Here's the drawing with two shaded views (mm, measured from the low corner). I have some questions. Give positions to 0.01 mm unless a question says otherwise; leave off trailing zeros. Loops run counter-clockwise (first coordinate to the right, second up) from the corner with the lowest first, then second, coordinate; pieces in that order, holes last. Notation, with made-up numbers: (60, 18.5) - (97, 18.5) arc R13 ccw to (97, 28.5) - close; hole circle Ø1 at (26.25, -5.75). An arc over 180 degrees is marked (long way). Use a Markdown table: item, result. Add a question column.
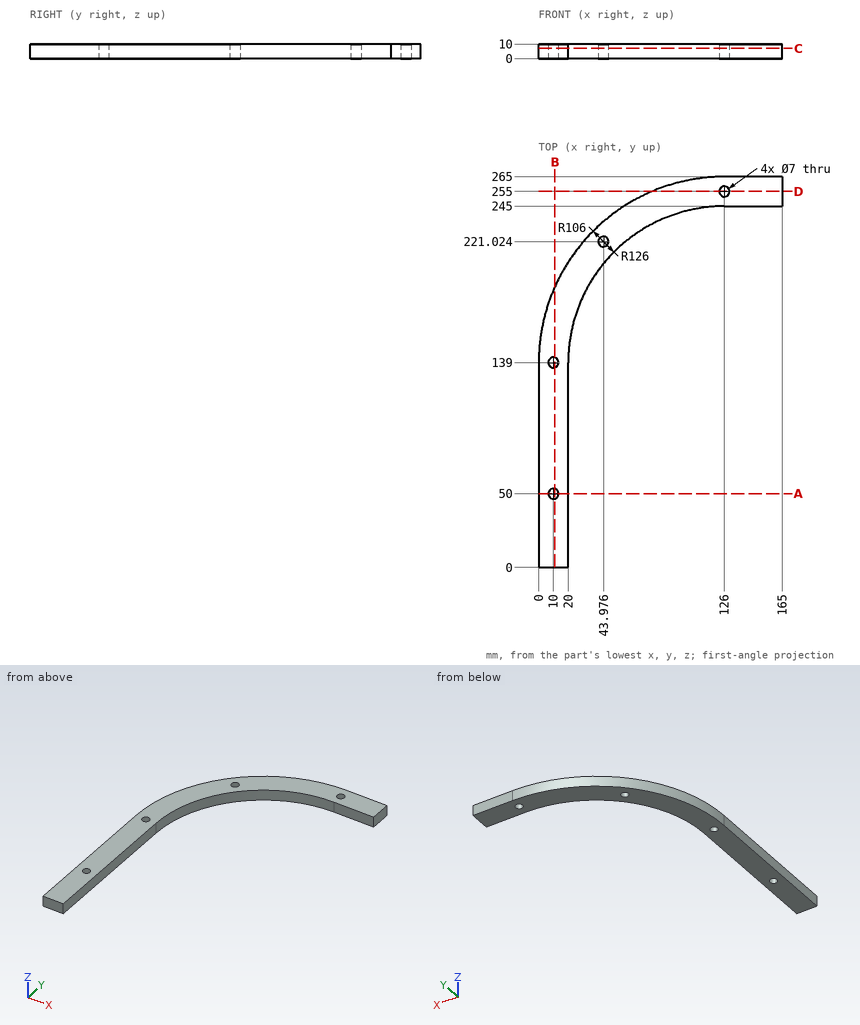
1. Suppose I cut it at B-B (x = 11). List the corners of the cut face in (y, z) for me, and give its area (3 significant figures).
2. Will these pins go through, and if not, where does the flat tip stop? P1, Ø11, axis at x = 126, y = 255, coming from the +Z side; P2, Ø5, axis at y = 188, z = 8.5, coming from the +X side; P3, Ø3, axis at y = 63.5, z = 7, coming from the +X side; P4, Ø3, axis at x = 139.5, z = 4, coming from the -Y side.
3. Please list where these lines run through material, in increasing order: line 1 along Y through (x, z) = (10, 4.5) (1 decimal); line 2 along X through (y, z) = (66, 5); line 3 along X through (y, z) = (139.5, 6.75) (1 decimal). Write a range as [from, to].
4. Suppose I cut it at A-A (y = 50). List the corners of the cut face in (x, z) for me.
5. Suppose I cut it at D-D (y = 255). List the corners of the cut face in (x, z) for me.
6. Suppose I cut it at C-C (z = 7). List the corners of the cut face in (x, y) for me (1 decimal).
Results below:
| question | item | result |
|---|---|---|
| 1 | outline | (0, 0) - (46.65, 0) - (46.65, 10) - (0, 10) - close; (53.35, 0) - (135.65, 0) - (135.65, 10) - (53.35, 10) - close; (142.35, 0) - (190.49, 0) - (190.49, 10) - (142.35, 10) - close |
| 1 | area | 1,770 mm² |
| 2 | P1 | z = 10 |
| 2 | P2 | x = 33.35 |
| 2 | P3 | x = 20 |
| 2 | P4 | y = 245 |
| 3 | line 1 | [0, 46.5], [53.5, 135.5], [142.5, 188.2] |
| 3 | line 2 | [0, 20] |
| 3 | line 3 | [0, 6.5], [13.5, 20] |
| 4 | outline | (0, 0) - (6.5, 0) - (6.5, 10) - (0, 10) - close; (13.5, 0) - (20, 0) - (20, 10) - (13.5, 10) - close |
| 5 | outline | (76.81, 0) - (122.5, 0) - (122.5, 10) - (76.81, 10) - close; (129.5, 0) - (165, 0) - (165, 10) - (129.5, 10) - close |
| 6 | outline | (0, 0) - (20, 0) - (20, 139) arc R106 cw to (126, 245) - (165, 245) - (165, 265) - (126, 265) arc R126 ccw to (0, 139) - close; hole circle Ø7 at (10, 50); hole circle Ø7 at (10, 139); hole circle Ø7 at (44, 221); hole circle Ø7 at (126, 255) |
